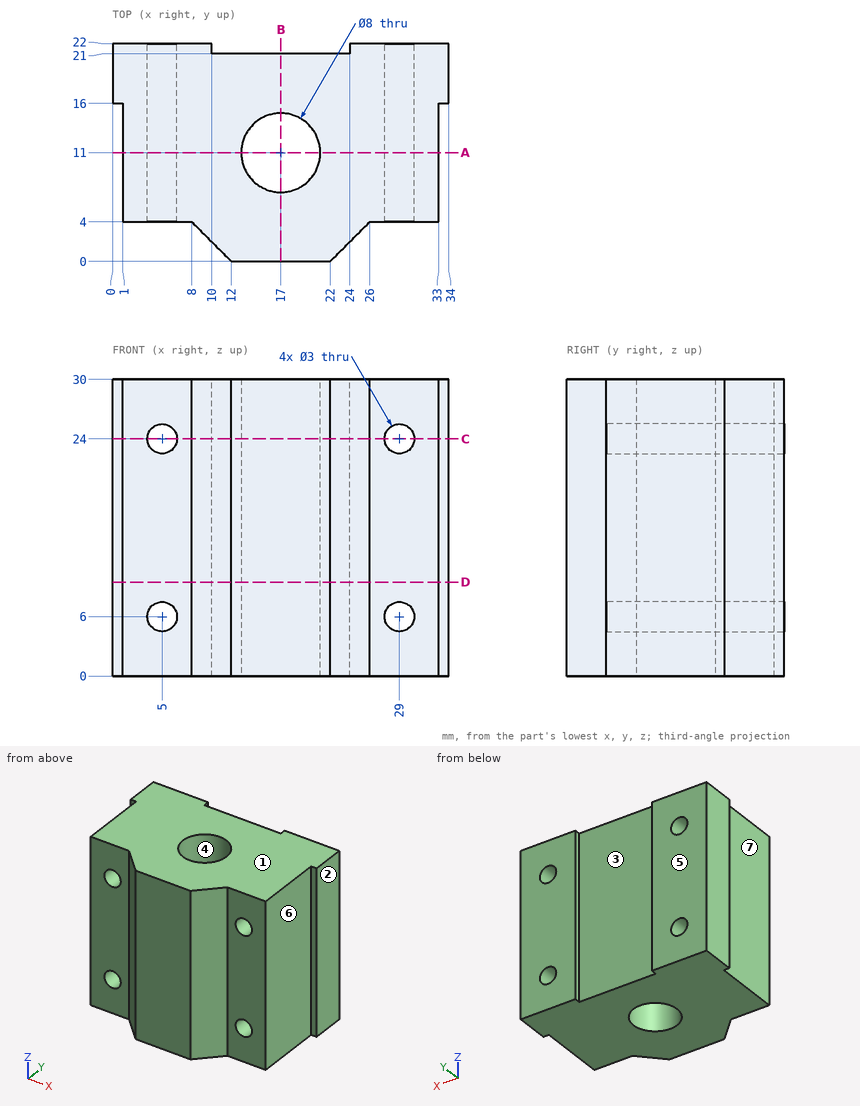
Geometry: see drawing. Coordinates: mm, zero at the bounding-box minimum. A direction names the side the tool comes from. Coordinates: 2 decimals unless noted, no trailing zeros. Write each loop counter-clockwise with the first axis right and the second up, starting at its lowest first coordinate (ties: lowest second). Pieces come first, ordered by that corner, then holes. Notation, with made-up numbers: M -36,88 L 10,88 A5 ccw 10,96 Z; hole C -1.5,-19.75 d8. An arc over 180 degrees is marked long. Answer as a JSON object with one key per item and string values.
1. Cut plane B-B on x = 17. Output: boundary loops of the cut face in (y, z), plus the area to 3 significant figures.
Evaluation:
{"outline": "M 0,0 L 7,0 L 7,30 L 0,30 Z; M 15,0 L 21,0 L 21,30 L 15,30 Z", "area": "390 mm^2"}
2. Contact query for flat-ended pins moving along their axis: P1, Ø1.5, axis at x = 23, z = 10.5, coming from the +Y side; P2, Ø3.5, axis at y = 9.5, z = 14.5, coming from the -X side; P3, Ø0.5, axis at x = 0.5, z = 20.5, coming from the -Y side. Output: stop coordinate, or through.
Evaluation:
{"P1": "y = 21", "P2": "x = 1", "P3": "y = 16"}
3. Cut plane D-D on z = 9.5. Output: boundary loops of the cut face in (x, y).
Evaluation:
{"outline": "M 0,16 L 1,16 L 1,4 L 8,4 L 12,0 L 22,0 L 26,4 L 33,4 L 33,16 L 34,16 L 34,22 L 24,22 L 24,21 L 10,21 L 10,22 L 0,22 Z; hole C 17,11 d8"}
4. Cut plane A-A on y = 11. Output: boundary loops of the cut face in (x, z).
Evaluation:
{"outline": "M 1,0 L 13,0 L 13,30 L 1,30 Z; M 21,0 L 33,0 L 33,30 L 21,30 Z; hole C 5,6 d3; hole C 5,24 d3; hole C 29,6 d3; hole C 29,24 d3"}
5. Cut plane C-C on z = 24. Output: boundary loops of the cut face in (x, y).
Evaluation:
{"outline": "M 0,16 L 1,16 L 1,4 L 3.5,4 L 3.5,22 L 0,22 Z; M 6.5,4 L 8,4 L 12,0 L 22,0 L 26,4 L 27.5,4 L 27.5,22 L 24,22 L 24,21 L 10,21 L 10,22 L 6.5,22 Z; M 30.5,4 L 33,4 L 33,16 L 34,16 L 34,22 L 30.5,22 Z; hole C 17,11 d8"}
6. Ray query, L1, parallel to X at y = 17, z = 6; L2, parallel to X at y = 14, z = 6; L3, parallel to Z at x = 4, y = 9.5. Return the intervals inside material, ascending.
Evaluation:
{"L1": "0 to 3.5, 6.5 to 27.5, 30.5 to 34", "L2": "1 to 3.5, 6.5 to 14.35, 19.65 to 27.5, 30.5 to 33", "L3": "0 to 4.88, 7.12 to 22.88, 25.12 to 30"}
7. Access query for the marked faces 5, 6 and 7. Directions: +Z, -Z, +X, -X, +Y, -Y. A direction counts if a zero-diameter tool reaches every point of the face in a straight line with its end or side. Return the directions, or none.
Evaluation:
{"face 5": "+Z, -Z, +X, -X, +Y", "face 6": "+Z, -Z, +X, -Y", "face 7": "+Z, -Z, -X, -Y"}
8. Draft query along X for the marked faces 1, 2, 3 and 4. Return one class per face: released by +X, released by -X, zero draft, split by the parting line, or undercut.
Evaluation:
{"face 1": "zero draft", "face 2": "released by +X", "face 3": "undercut", "face 4": "undercut"}
